The listing builds one solid part. Answer for the finished solid, in the listing's coordinates (mm). Face numbers are marked on the shaded views. A direction names the side the tool comes from. Coordinates: 2 decimals unless noted, no trailing zeros. Order: outer loops, then holes, each group sorted by start corner. A loop starts at its lowest first (then second) coordinate and runs counter-clockwise, first axis right, second up. Notation, with made-up numbers: (14.25, 4) -> (49.25, 4) arc R28 cw to (49.25, 37) -> close; hole circle Ø10 at (18, 80.25). An arc over 180 degrees is marked (long way). Write item = value, one per line.
from build123d import *

# Parameters (mm, degrees)
SKETCH1_R           = 4.7625
BOSS_EXTRUDE1_DEPTH = 15
CUT_EXTRUDE1_DEPTH  = 66.383484153


with BuildPart() as part:
    # Sketch1 → Boss-Extrude1 (new body)
    with BuildSketch(Plane(origin=(0, 0, 0), x_dir=(1, 0, 0), z_dir=(0, 1, 0))):
        with BuildLine():
            Line((-31.819805153, 31.819805153), (-7.071067812, 7.071067812))
            ThreePointArc((-7.071067812, 7.071067812), (0, 10), (7.071067812, 7.071067812))
            Line((7.071067812, 7.071067812), (31.819805153, 31.819805153))
            ThreePointArc((31.819805153, 31.819805153), (0, -45), (-31.819805153, 31.819805153))
        make_face()
        with Locations(Location((0, 0, 0), (0, 0, 270))):
            Circle(SKETCH1_R, mode=Mode.SUBTRACT)
    extrude(amount=BOSS_EXTRUDE1_DEPTH)

    # Sketch4 → Cut-Extrude1 (cut, through all)
    with BuildSketch(Plane(origin=(0, 15, 0), x_dir=(1, 0, 0), z_dir=(0, 1, 0))):
        with BuildLine():
            Line((11.490666647, -9.641814145), (45.503789868, 30.893447649))
            ThreePointArc((45.503789868, 30.893447649), (34.992750198, -42.432386612), (-38.992939572, -38.788537785))
            Line((-38.992939572, -38.788537785), (11.490666647, -9.641814145))
        make_face()
    extrude(amount=-CUT_EXTRUDE1_DEPTH, mode=Mode.SUBTRACT)


solid = part.part
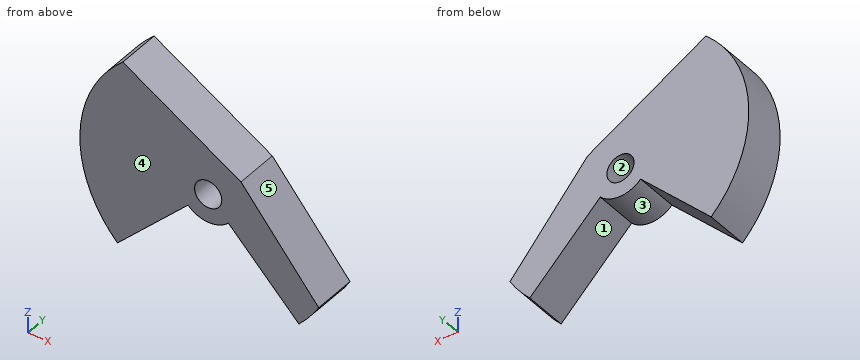
Q1. The mould has two halves that part along X. Classify the marked faces 3, 4 and 5: released by +X, released by -X, zero draft, split by the parting line, or undercut.
The answers:
face_3 = undercut
face_4 = zero draft
face_5 = released by +X
Q2. Section D-D, the plane x = 23.5 is taken. Give the vertices of the cut face in (y, z), plus the area to 3 significant figures.
The answers:
outline = (0, -23.5) -> (15, -23.5) -> (15, -4.67) -> (0, -4.67) -> close
area = 282 mm2
Q3. Section B-B, the plane z = -1.5 is taken. Give the vertices of the cut face in (x, y) (3 decimals), plus the area to 3 significant figures.
The answers:
outline = (-44.975, 0) -> (-4.52, 0) -> (-4.52, 15) -> (-44.975, 15) -> close; (4.52, 0) -> (20.84, 0) -> (20.84, 15) -> (4.52, 15) -> close
area = 852 mm2
Q4. Section C-C, the plane x = 0 is taken. Give the vertices of the cut face in (y, z).
The answers:
outline = (0, -10) -> (15, -10) -> (15, -4.76) -> (0, -4.76) -> close; (0, 4.76) -> (15, 4.76) -> (15, 16.28) -> (0, 16.28) -> close
Q5. Each of these flat-tipped pins is pushed along its axis until it touches: pin 1 Ø1.5 at (y, z) = (4, 5) entering from -X; pin 2 Ø8 at (x, y) = (-15.5, 12.5) entering from +Z; pin 3 Ø1.5 at (y, z) = (4.5, -11) entering from -X. Where does it stop, or does it pass through?
The answers:
pin_1 = -44.8
pin_2 = 27.53
pin_3 = -43.82
Q6. A tool of negligible diameter and unlimited length cuts with its end or side. For the marked faces 1 and 2, from which of +Z, -Z, +X, -X, +Y, -Y can it reach the whole face along a straight path? Write none if from no direction.
The answers:
face_1 = -Z, +Y, -Y
face_2 = +Y, -Y
Q7. Find the intervals of material crossed by line 1 along X through (y, z) = (8.5, 0); line 2 along Z through (x, y) = (1, 12.5); line 3 along X through (y, z) = (2.25, 14), in increasing order.
The answers:
line_1 = -45 to -4.76, 4.76 to 19.58
line_2 = -9.95 to -4.66, 4.66 to 15.7
line_3 = -42.77 to 3.94
Q8. Section A-A, the plane y = 6 is taken. Give the vertices of the cut face in (x, z) (1 decimal), plus the area to 3 significant figures.
The answers:
outline = (-31.8, -31.8) -> (-7.1, -7.1) arc R10 ccw to (7.1, -7.1) -> (31.8, -31.8) arc R45 ccw to (38.8, -22.9) -> (11.5, 9.6) -> (-30, 33.6) arc R45 ccw to start; hole circle Ø9.5 at (0, 0)
area = 2,570 mm2
